from build123d import *

# Parameters (mm, degrees)
SKETCH2_R                                      = 12.7
BOSS_EXTRUDE6_DEPTH                            = 40.64
SKETCH3_R                                      = 3.5
CUT_EXTRUDE1_DEPTH                             = 40.64
SKETCH4_R                                      = 1.778
CUT_EXTRUDE2_DEPTH                             = 6
BOSS_EXTRUDE8_DEPTH                            = 10
SKETCH8_W                                      = 25.185693912
SKETCH8_H                                      = 10
BOSS_EXTRUDE9_DEPTH                            = 7.284789049
BOSS_EXTRUDE10_DEPTH                           = 30.64
CSK_FOR_M3_FLAT_HEAD_MACHINE_SCREW1_AT_2_COUNT = 2
CSK_FOR_M3_FLAT_HEAD_MACHINE_SCREW1_AT_2_PITCH = 9.039543014
CSK_FOR_M3_FLAT_HEAD_MACHINE_SCREW1_AT_3_COUNT = 2
CSK_FOR_M3_FLAT_HEAD_MACHINE_SCREW1_AT_3_PITCH = 9.039543014
SKETCH16_W                                     = 3.769994858
SKETCH16_H                                     = 22.000968128
CUT_EXTRUDE3_DEPTH                             = 25
SKETCH17_W                                     = 10.276759259
SKETCH17_H                                     = 15.64
CUT_EXTRUDE4_DEPTH                             = 2.743753899
SKETCH18_W                                     = 12.6
SKETCH18_H                                     = 15.64
CUT_EXTRUDE5_DEPTH                             = 2.743753899


with BuildPart() as part:
    # Sketch2 → Boss-Extrude6 (new body)
    with BuildSketch(Plane(origin=(0, -2111.389926236, 0), x_dir=(1, 0, 0), z_dir=(0, 1, 0))):
        with Locations(Location((-53.693967541, 163.840329354, 0), (0, 0, 180))):
            Circle(SKETCH2_R)
    extrude(amount=BOSS_EXTRUDE6_DEPTH)

    # Sketch3 → Cut-Extrude1 (cut)
    with BuildSketch(Plane(origin=(0, -2070.749926236, 0), x_dir=(1, 0, 0), z_dir=(0, 1, 0))):
        with Locations(Location((-53.693967541, 163.840329354, 0), (0, 0, 270))):
            Circle(SKETCH3_R)
    extrude(amount=-CUT_EXTRUDE1_DEPTH, mode=Mode.SUBTRACT)

    # Sketch4 → Cut-Extrude2 (cut)
    with BuildSketch(Plane.XZ.offset(2111.389926236)):
        with Locations(Location((-61.942859512, -159.077829354, 0), (0, 0, 270))):
            Circle(SKETCH4_R)
        with Locations(Location((-53.693967541, -173.365329354, 0), (0, 0, 270))):
            Circle(SKETCH4_R)
        with Locations(Location((-45.44507557, -159.077829354, 0), (0, 0, 270))):
            Circle(SKETCH4_R)
    extrude(amount=-CUT_EXTRUDE2_DEPTH, mode=Mode.SUBTRACT)

    # Sketch7 → Boss-Extrude8 (add)
    with BuildSketch(Plane.XZ.offset(2111.389926236)):
        with BuildLine():
            Line((-40.993967541, -163.840329354), (-40.993967541, -182.634287878))
            Line((-40.993967541, -182.634287878), (-66.179661453, -182.634287878))
            Line((-66.179661453, -182.634287878), (-66.179661453, -166.163570095))
            ThreePointArc((-66.179661453, -166.163570095), (-52.527415502, -176.486639343), (-40.993967541, -163.840329354))
        make_face()
    extrude(amount=-BOSS_EXTRUDE8_DEPTH)

    # Sketch8 → Boss-Extrude9 (add)
    with BuildSketch(Plane(origin=(0, 0, -182.634287878), x_dir=(-1, 0, 0), z_dir=(0, 0, -1))):
        with Locations((53.586814497, -2106.389926236)):
            Rectangle(SKETCH8_W, SKETCH8_H)
    extrude(amount=BOSS_EXTRUDE9_DEPTH)

    # Sketch9 → Boss-Extrude10 (add)
    with BuildSketch(Plane(origin=(0, -2070.749926236, 0), x_dir=(1, 0, 0), z_dir=(0, 1, 0))):
        with BuildLine():
            Line((-66.179661453, 163.840329354), (-66.179661453, 189.919076927))
            Line((-66.179661453, 189.919076927), (-40.993967541, 189.919076927))
            Line((-40.993967541, 189.919076927), (-40.993967541, 163.840329354))
            ThreePointArc((-40.993967541, 163.840329354), (-53.586814497, 176.43317631), (-66.179661453, 163.840329354))
        make_face()
    extrude(amount=-BOSS_EXTRUDE10_DEPTH)

    # Sketch15 → CSK for M3 Flat Head Machine Screw1 (revolve, cut)
    with BuildSketch(Plane(origin=(-53.586814498, -2075.749926236, -189.919076927), x_dir=(0, 1, 0), z_dir=(1, 0, 0))):
        Polygon((0, 0), (0, 10), (1.7, 8.978536948), (1.7, 1.45), (3.15, 0), align=None)
    csk_for_m3_flat_head_machine_screw1 = revolve(axis=Axis((-53.586814498, -2075.749926236, -196.269076927), (0, 0, 1)), mode=Mode.SUBTRACT)

    # CSK for M3 Flat Head Machine Screw1 at 2: CSK for M3 Flat Head Machine Screw1 ×2
    with Locations(*[(-i * CSK_FOR_M3_FLAT_HEAD_MACHINE_SCREW1_AT_2_PITCH, 0, 0) for i in range(1, CSK_FOR_M3_FLAT_HEAD_MACHINE_SCREW1_AT_2_COUNT)]):
        add(csk_for_m3_flat_head_machine_screw1, mode=Mode.SUBTRACT)

    # CSK for M3 Flat Head Machine Screw1 at 3: CSK for M3 Flat Head Machine Screw1 ×2
    with Locations(*[(i * CSK_FOR_M3_FLAT_HEAD_MACHINE_SCREW1_AT_3_PITCH, 0, 0) for i in range(1, CSK_FOR_M3_FLAT_HEAD_MACHINE_SCREW1_AT_3_COUNT)]):
        add(csk_for_m3_flat_head_machine_screw1, mode=Mode.SUBTRACT)

    # Mirror1: CSK for M3 Flat Head Machine Screw1 across plane
    add(csk_for_m3_flat_head_machine_screw1.mirror(Plane.ZX.offset(-2091.069926234)), mode=Mode.SUBTRACT)

    # Mirror1 copy 1 sketch → Mirror1 copy 1 (revolve, cut)
    with BuildSketch(Plane(origin=(-62.626357512, -2106.389926232, -189.919076927), x_dir=(0, -1, 0), z_dir=(1, 0, 0))):
        Polygon((0, 0), (0, -10), (1.7, -8.978536948), (1.7, -1.45), (3.15, 0), align=None)
    revolve(axis=Axis((-62.626357512, -2106.389926232, -196.269076927), (0, 0, -1)), mode=Mode.SUBTRACT)

    # Mirror1 copy 2 sketch → Mirror1 copy 2 (revolve, cut)
    with BuildSketch(Plane(origin=(-44.547271484, -2106.389926232, -189.919076927), x_dir=(0, -1, 0), z_dir=(1, 0, 0))):
        Polygon((0, 0), (0, -10), (1.7, -8.978536948), (1.7, -1.45), (3.15, 0), align=None)
    revolve(axis=Axis((-44.547271484, -2106.389926232, -196.269076927), (0, 0, -1)), mode=Mode.SUBTRACT)

    # Sketch16 → Cut-Extrude3 (cut)
    with BuildSketch(Plane(origin=(0, -2070.749926236, 0), x_dir=(1, 0, 0), z_dir=(0, 1, 0))):
        with Locations((-65.320904983, 165.43984529)):
            Rectangle(SKETCH16_W, SKETCH16_H)
        with Locations((-41.852724011, 165.43984529)):
            Rectangle(SKETCH16_W, SKETCH16_H)
    extrude(amount=-CUT_EXTRUDE3_DEPTH, mode=Mode.SUBTRACT)

    # Sketch17 → Cut-Extrude4 (cut)
    with BuildSketch(Plane.ZY.offset(66.179661453)):
        with Locations((-171.301949724, -2103.569926236)):
            Rectangle(SKETCH17_W, SKETCH17_H)
    extrude(amount=-CUT_EXTRUDE4_DEPTH, mode=Mode.SUBTRACT)

    # Sketch18 → Cut-Extrude5 (cut)
    with BuildSketch(Plane(origin=(-40.993967541, 0, 0), x_dir=(0, 0, -1), z_dir=(1, 0, 0))):
        with Locations((170.140329354, -2103.569926236)):
            Rectangle(SKETCH18_W, SKETCH18_H)
    extrude(amount=-CUT_EXTRUDE5_DEPTH, mode=Mode.SUBTRACT)


solid = part.part
Geometry check sheet. Reference: the model listing, model coordinates, mm. A direction names the side the tool comes from. Give positions to 0.01 mm unless a question says otherwise; leave off trailing zeros. Write each loop counter-clockwise with the first axis right and the second up, starting at its lowest first coordinate (ties: lowest second). Pieces come first, ordered by that corner, then holes. Notation, with made-up numbers: M -26.5,0 L 16.5,0 A27 cw 16.5,24 Z; hole C 60.5,2 d11. An arc over 180 degrees is marked long. Answer as CSV lines item,"result". Start each with the question number.
Q1. Section check B-B, the plane z = -158.5. Record the cut outline in (x, y), then the cut area to 3 significant figures.
Q2. Go/stop test with flat-tipped pins: pin 1 (1.4 mm diameter, centred on x = -64.5, y = -2084.5, fed in from +Z); pin 2 (4 mm diameter, centred on x = -62.63, y = -2106.39, fed in from +Z); pin 3 (23 mm diameter, centred on y = -2083, z = -166.5, fed in from -X). Record where each tip stops, or that it passes through.
Q3. Material ranges on L1, parallel to X at y = -2106.5, z = -181; L2, parallel to X at y = -2073.5, z = -187; L3, parallel to Z at x = -64, y = -2093, recorded low to high.
Q4. Tool access check on faces 4 (the face through (-42, -2104, -163.84)), 5 (the face through (-45, -2105.39, -159)), 6 (the face through (-65, -2104, -166.164)), 7 (the face through (-63.436, -2086, -166)), 8 (the face through (-53.66, -2077.45, -184.76)). Record the directions out of +Z, -Z, +X, -X, +Y, -Y that give a thin tool (end or side, any length) a straight path to the whole face; none if there is none.
Q5. Section check C-C, the plane y = -2080. Record the cut outline in (x, z), then the cut area to 3 significant figures.
Q6. Section check A-A, the plane y = -2099.5. Record the cut outline in (x, z).
Q7. Section check D-D, the plane z = -171. Record the cut outline in (x, y).
Q8. Release check for a two-part mould opening along Z. For faces 1 (the face through (-65, -2095.75, -162)), 2 (the face through (-62, -2105.39, -159)), 3 (the face through (-62.715, -2106.672, -180.096)) record: pulls with the +Z half, pulls with the -Z half, needs draft (parallel to the pull), parting line crosses it, or undercut.
Geometry says:
1,outline,"M -65.22,-2111.39 L -63.62,-2111.39 L -63.62,-2105.39 L -60.26,-2105.39 L -60.26,-2111.39 L -47.13,-2111.39 L -47.13,-2105.39 L -43.76,-2105.39 L -43.76,-2111.39 L -42.17,-2111.39 L -42.17,-2095.75 L -43.74,-2095.75 L -43.74,-2070.75 L -63.44,-2070.75 L -63.44,-2095.75 L -65.22,-2095.75 Z"
1,area,"813 mm^2"
2,pin 1,"z = -176.44"
2,pin 2,"z = -153.2"
2,pin 3,"x = -66.18"
3,L1,"-66.18 to -64.32, -60.93 to -55.28, -51.89 to -46.24, -42.85 to -40.99"
3,L2,"-66.18 to -40.99"
3,L3,"-189.92 to -176.44"
4,face 4,"+X, +Y, -Y"
4,face 5,"-Y"
4,face 6,"-X, +Y, -Y"
4,face 7,"-X, +Y"
4,face 8,"-Z"
5,outline,"M -66.18,-189.92 L -40.99,-189.92 L -40.99,-176.44 L -43.74,-176.44 L -43.74,-155.96 A12.7 ccw -63.44,-155.69 L -63.44,-176.44 L -66.18,-176.44 Z; hole C -53.69,-163.84 d7"
5,area,"771 mm^2"
6,outline,"M -66.18,-189.92 L -40.99,-189.92 L -40.99,-176.44 L -43.74,-176.44 L -43.74,-163.84 L -40.99,-163.84 A12.7 ccw long -66.18,-166.16 L -63.44,-166.16 L -63.44,-176.44 L -66.18,-176.44 Z; hole C -53.69,-163.84 d7"
7,outline,"M -63.44,-2111.39 L -43.74,-2111.39 L -43.74,-2070.75 L -63.44,-2070.75 Z"
8,face 1,"needs draft"
8,face 2,"undercut"
8,face 3,"pulls with the -Z half"
